Geometry: final body of the model. Coordinates: model frame, mm. A direction names the side the tool comes from. Give positions to 0.01 mm unless a question says otherwise; leave off trailing zeros. Order: outer loops, then holes, each group sorted by start corner. A loop starts at its lowest first (then second) coordinate and runs counter-clockwise, first axis right, second up. Notation, with made-up numbers: (66.25, 40) -> (100.25, 40) arc R22 ccw to (100.25, 74) -> close; hole circle Ø3 at (7.5, -2.75). An arc over 180 degrees is marked (long way). One line per question, with ' | ' between items. Start each with the question number.
(1) Mould query, pull axis X, two halves, no side actions, for faces 4 (the face through (-148, -38.1, -3)), 5 (the face through (0, -50, -3)), 6 (the face through (-20, 0, -3)). Classes: +X half, -X half, draft (parallel to the pull), parting line (faces both ways), or undercut.
(2) First-contact query: pin 1 Ø1.7 at (x, z) = (-15.5, -2.5) entering from -Y; pin 2 Ø2.5 at (x, z) = (-136.5, -2) entering from +Y. Flat tips, straight axial feed; report the tip coordinate or a pass-through.
(3) Section D-D (z = -4.75). State how many separate pieces and enclosed holes the cut face has, then the cut area to 3 significant figures.
(4) Section C-C (y = -17.78). Return loops of the section in (x, z).
(5) Ray query, L1, parallel to Y at x = -19.05, z = -2; L2, parallel to X at y = -45.5, z = -2.5; L3, parallel to X at y = -95, z = -4.5. Return the intervals inside material, ascending.
(6) Section A-A (x = -95.25). Return loops of the section in (y, z), then the cut area to 3 significant figures.
(7) Set-up query: faces 1 (the face through (-10.846, -91, -3)), 2 (the face through (-1.588, -51, -3)), 3 (the face through (-10.846, -3, -3)). Return all of +Z, -Z, +X, -X, +Y, -Y with unobstructed straight access to the full face (end or side cutting, diameter ignored); none if empty.
(8) Section B-B (y = -45). Return loops of the section in (x, z).
Autodesk Inventor part; units mm, degrees
ref_plane "Work Plane1" through (0, 0, 0) normal (0, 0, 1) x (1, 0, 0)
ref_plane "Work Plane2" through (-137.8458, 0, 0) normal (0, 1, 0) x (1, 0, 0)
ref_plane "YZ Plane" through (0, 0, 0) normal (1, 0, 0) x (0, 1, 0)
ref_plane "Work Plane1" through (0, 0, 0) normal (0, 0, 1) x (1, 0, 0)
sketch "Sketch1" plane through (0, 0, 0) normal (0, 0, 1) x (1, 0, 0)
  line L0 (-77.8391, 0) -> (-108.8361, 0)
  line L1 (-108.8361, -33.02) -> (-108.8361, 0)
  line L2 (-77.8391, -33.02) -> (-108.8361, -33.02)
  line L3 (-77.8391, -33.02) -> (-77.8391, 0)
  line L4 (-152.4, 0) -> (0, 0) construction
  line L5 (-152.4, 0) -> (-152.4, 6.35) construction
  line L6 (0, 0) -> (0, 6.35) construction
  line L7 (-152.4, 0) -> (0, 0)
  line L8 (0, 0) -> (0, -101.6)
  line L9 (0, -101.6) -> (-152.4, -101.6)
  line L10 (-152.4, -101.6) -> (-152.4, 0)
  line L11 (-137.8458, 6.35) -> (-137.8458, 0)
  line L12 (-141.5542, 6.35) -> (-141.5542, 0)
  line L13 (-14.5542, 6.35) -> (-14.5542, 0)
  line L14 (-10.8458, 6.35) -> (-10.8458, 0)
  line L15 (-141.5542, 0) -> (-137.8458, 0)
  line L16 (-137.8458, 0) -> (-137.8458, -12.7)
  line L17 (-137.8458, -12.7) -> (-141.5542, -12.7)
  line L18 (-141.5542, -12.7) -> (-141.5542, 0)
  line L19 (-14.5542, 0) -> (-10.8458, 0)
  line L20 (-10.8458, 0) -> (-10.8458, -12.7)
  line L21 (-10.8458, -12.7) -> (-14.5542, -12.7)
  line L22 (-14.5542, -12.7) -> (-14.5542, 0)
  line L23 (-16.637, -5.7726) -> (-8.763, -5.7726)
  line L24 (-8.763, -5.7726) -> (-8.763, -8.5666)
  line L25 (-8.763, -8.5666) -> (-16.637, -8.5666)
  line L26 (-16.637, -8.5666) -> (-16.637, -5.7726)
  line L27 (-143.637, -5.7726) -> (-135.763, -5.7726)
  line L28 (-135.763, -5.7726) -> (-135.763, -8.5666)
  line L29 (-135.763, -8.5666) -> (-143.637, -8.5666)
  line L30 (-143.637, -8.5666) -> (-143.637, -5.7726)
  line L31 (-152.4, -50.8) -> (0, -50.8) construction
  line L32 (-137.8458, -107.95) -> (-137.8458, -101.6)
  line L33 (-141.5542, -107.95) -> (-141.5542, -101.6)
  line L34 (-14.5542, -107.95) -> (-14.5542, -101.6)
  line L35 (-10.8458, -107.95) -> (-10.8458, -101.6)
  line L36 (-141.5542, -101.6) -> (-137.8458, -101.6)
  line L37 (-137.8458, -101.6) -> (-137.8458, -88.9)
  line L38 (-137.8458, -88.9) -> (-141.5542, -88.9)
  line L39 (-141.5542, -88.9) -> (-141.5542, -101.6)
  line L40 (-14.5542, -101.6) -> (-10.8458, -101.6)
  line L41 (-10.8458, -101.6) -> (-10.8458, -88.9)
  line L42 (-10.8458, -88.9) -> (-14.5542, -88.9)
  line L43 (-14.5542, -88.9) -> (-14.5542, -101.6)
  line L44 (-16.637, -95.8274) -> (-8.763, -95.8274)
  line L45 (-8.763, -95.8274) -> (-8.763, -93.0334)
  line L46 (-8.763, -93.0334) -> (-16.637, -93.0334)
  line L47 (-16.637, -93.0334) -> (-16.637, -95.8274)
  line L48 (-143.637, -95.8274) -> (-135.763, -95.8274)
  line L49 (-135.763, -95.8274) -> (-135.763, -93.0334)
  line L50 (-135.763, -93.0334) -> (-143.637, -93.0334)
  line L51 (-143.637, -93.0334) -> (-143.637, -95.8274)
  dimension "d0" = 101.6
  dimension "d1" = 12.7
  dimension "d2" = 7.874
  dimension "d3" = 2.794
  dimension "d6" = 2.0828
  dimension "d7" = 2.0828
  dimension "d8" = 7.874
  dimension "d9" = 2.0828
  dimension "d10" = 2.0828
ref_plane "Work Plane2" through (-137.8458, 0, 0) normal (0, 1, 0) x (1, 0, 0)
sketch "Sketch2" plane through (-137.8458, 0, 0) normal (0, 1, 0) x (1, 0, 0)
  line L0 (35.8892, 0) -> (10.4892, 0)
  line L1 (10.4892, 0) -> (10.4892, 6.35)
  line L2 (10.4892, 6.35) -> (35.8892, 6.35)
  line L3 (35.8892, 6.35) -> (35.8892, 0)
  line L4 (112.0892, 0) -> (86.6892, 0)
  line L5 (112.0892, 6.35) -> (112.0892, 0)
  line L6 (86.6892, 6.35) -> (112.0892, 6.35)
  line L7 (86.6892, 0) -> (86.6892, 6.35)
  point P0 (137.8458, 0)
extrude "Extrusion2" add sketch "Sketch2" along normal blind 6.35
extrude "Extrusion3" add sketch "Sketch1" against normal blind 6.35 contours L3 L2 L1 L0 | L7 L22 L23 L26 L25 L21 L20 L24 L8 L9 L41 L44 L45 L46 L42 L43 L47 L37 L48 L49 L50 L38 L39 L51 L10 L18 L27 L30 L29 L17 L16 L28 L1 L2 L3
sketch "Sketch3" plane through (-137.8458, -101.6, 0) normal (0, -1, 0) x (1, 0, 0)
  line L0 (35.8892, 0) -> (35.8892, -6.35)
  line L1 (35.8892, -6.35) -> (10.4892, -6.35)
  line L2 (10.4892, -6.35) -> (10.4892, 0)
  line L3 (10.4892, 0) -> (35.8892, 0)
  line L4 (112.0892, 0) -> (112.0892, -6.35)
  line L5 (112.0892, -6.35) -> (86.6892, -6.35)
  line L6 (86.6892, -6.35) -> (86.6892, 0)
  line L7 (86.6892, 0) -> (112.0892, 0)
  point P0 (137.8458, 0)
extrude "Extrusion4" add sketch "Sketch3" along normal blind 6.35
sketch "Sketch4" plane through (-101.9566, 6.35, -6.35) normal (0, 0, -1) x (-1, 0, 0)
  line L0 (48.8559, -69.85) -> (48.8559, -44.45)
  line L1 (48.8559, -44.45) -> (42.5059, -44.45)
  line L2 (42.5059, -44.45) -> (42.5059, -69.85)
  line L3 (42.5059, -69.85) -> (48.8559, -69.85)
extrude "Extrusion5" cut sketch "Sketch4" against normal through all
ref_plane "Work Plane3" through (-76.2, -101.6, 0) normal (-1, 0, 0) x (0, 0, 1)
mirror "Mirror1" about plane through (-76.2, -101.6, 0) normal (-1, 0, 0) of "Extrusion5"
sketch "Sketch5" plane through (-101.9566, 6.35, -6.35) normal (0, 0, -1) x (-1, 0, 0)
  line L0 (0, -6.35) -> (-50.8, -6.35)
  line L1 (-101.9566, -6.35) -> (-101.9566, -107.95)
  line L2 (50.4434, -107.95) -> (50.4434, -6.35)
  line L3 (35.8892, -6.35) -> (25.4, -6.35)
  circle A0 centre (31.3934, -24.13) radius 3.9688
  circle A1 centre (-6.7066, -24.13) radius 3.9688
  circle A2 centre (-44.8066, -24.13) radius 3.9688
  circle A3 centre (-82.9066, -24.13) radius 3.9688
  circle A4 centre (31.3934, -62.23) radius 3.9688
  circle A5 centre (-6.7066, -62.23) radius 3.9688
  circle A6 centre (-44.8066, -62.23) radius 3.9688
  circle A7 centre (-82.9066, -62.23) radius 3.9688
  dimension "d21" = 7.9375
  dimension "d22" = 17.78
  dimension "d25" = 38.1
  dimension "d30" = 19.05
  dimension "d31" = 19.05
  dimension "d34" = 38.1
extrude "Extrusion6" cut sketch "Sketch5" against normal through all
equation "\"d6\" = d7"
equation "\"d9\" = d10"
equation "\"d30\" = d31"
properties part number "baseBoxShortSideRB02"
Response:
1) face 4: undercut | face 5: +X half | face 6: draft
2) pin 1: stops at y = -101.6 | pin 2: stops at y = 0
3) separate pieces: 1 | enclosed holes: 10 | area: 15,200 mm^2
4) outline: (-152.4, -6.35) -> (-137.32, -6.35) -> (-137.32, 0) -> (-152.4, 0) -> close; (-129.38, -6.35) -> (-99.22, -6.35) -> (-99.22, 0) -> (-129.38, 0) -> close; (-91.28, -6.35) -> (-61.12, -6.35) -> (-61.12, 0) -> (-91.28, 0) -> close; (-53.18, -6.35) -> (-23.02, -6.35) -> (-23.02, 0) -> (-53.18, 0) -> close; (-15.08, -6.35) -> (0, -6.35) -> (0, 0) -> (-15.08, 0) -> close
5) L1: y = -101.6 to -59.85, -51.91 to -21.75, -13.81 to 0 | L2: x = -152.4 to -150.81, -144.46 to -7.94, -1.59 to 0 | L3: x = -152.4 to -143.64, -135.76 to -16.64, -8.76 to 0
6) outline: (-101.6, -6.35) -> (-59.85, -6.35) -> (-59.85, 0) -> (-101.6, 0) -> close; (-51.91, -6.35) -> (-21.75, -6.35) -> (-21.75, 0) -> (-51.91, 0) -> close; (-13.81, -6.35) -> (0, -6.35) -> (0, 0) -> (-13.81, 0) -> close | area: 544 mm^2
7) face 1: +Z, -Z, -Y | face 2: +Z, -Z | face 3: +Z, -Z, +Y
8) outline: (-152.4, -6.35) -> (-150.81, -6.35) -> (-150.81, 0) -> (-152.4, 0) -> close; (-144.46, -6.35) -> (-7.94, -6.35) -> (-7.94, 0) -> (-144.46, 0) -> close; (-1.59, -6.35) -> (0, -6.35) -> (0, 0) -> (-1.59, 0) -> close
